Work out the finished part from the listing and answer in its coordinate system (mm). Coordinates: 2 decimals unless noted, no trailing zeros. Order: outer loops, then holes, each group sorted by start corner. A loop starts at its lowest first (then second) coordinate and runs counter-clockwise, first axis right, second up. Notation, with made-up numbers: (62, -29) -> (94, -29) arc R23 cw to (94, -2) -> close; hole circle Ø9 at (76, 83). An arc over 180 degrees is marked (long way). Use one line per item in the form item = value.
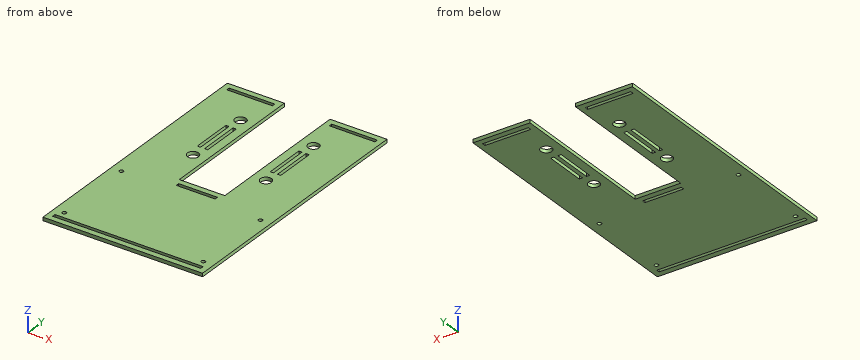
Autodesk Inventor part; units mm, degrees
ref_plane "YZ Plane" through (0, 0, 0) normal (1, 0, 0) x (0, 1, 0)
ref_plane "XZ Plane" through (0, 0, 0) normal (0, 1, 0) x (-1, 0, 0)
ref_plane "XY Plane" through (0, 0, 0) normal (0, 0, 1) x (1, 0, 0)
sketch "Sketch1" plane through (0, 0, 0) normal (0, 0, 1) x (1, 0, 0)
  line L0 (0, 0) -> (140, 0)
  line L1 (140, 0) -> (140, 232.6)
  line L2 (140, 232.6) -> (90, 232.6)
  line L3 (90, 232.6) -> (90, 100)
  line L4 (90, 100) -> (50, 100)
  line L5 (50, 100) -> (50, 232.6)
  line L6 (50, 232.6) -> (0, 232.6)
  line L7 (0, 232.6) -> (0, 0)
  line L8 (70, 100) -> (70, 0) construction
  line L9 (30, 232.2963) -> (30, 0) construction
  circle A0 centre (38, 194.6) radius 4.85
  circle A1 centre (38, 134.6) radius 4.85
  circle A2 centre (102, 194.6) radius 4.85
  circle A3 centre (102, 134.6) radius 4.85
  circle A4 centre (30, 194.6) radius 14 construction
  circle A5 centre (30, 134.6) radius 14 construction
  line L10 (5, 227.6) -> (45, 227.6)
  line L11 (45, 227.6) -> (45, 224.6)
  line L12 (45, 224.6) -> (5, 224.6)
  line L13 (5, 224.6) -> (5, 227.6)
  line L14 (53, 95) -> (87, 95)
  line L15 (87, 95) -> (87, 92)
  line L16 (87, 92) -> (53, 92)
  line L17 (53, 92) -> (53, 95)
  line L18 (5, 8) -> (135, 8)
  line L19 (135, 8) -> (135, 5)
  line L20 (135, 5) -> (5, 5)
  line L21 (5, 5) -> (5, 8)
  line L22 (135, 227.6) -> (95, 227.6)
  line L23 (95, 227.6) -> (95, 224.6)
  line L24 (95, 224.6) -> (135, 224.6)
  line L25 (135, 224.6) -> (135, 227.6)
  line L26 (30, 194.6) -> (50, 194.6) construction
  line L27 (30, 134.6) -> (50, 134.6) construction
  circle A6 centre (30, 202.6) radius 4.5
  dimension "d0" = 40
  dimension "d2" = 132.6
  dimension "d3" = 100
  dimension "d4" = 9.7
  dimension "d6" = 60
  dimension "d10" = 28
  dimension "d11" = 8
  dimension "d12" = 8
  dimension "d13" = 5
  dimension "d14" = 5
  dimension "d15" = 5
  dimension "d16" = 3
  dimension "d17" = 3
  dimension "d18" = 5
  dimension "d19" = 3
  dimension "d20" = 3
  dimension "d21" = 5
  dimension "d22" = 5
  dimension "d23" = 5
  dimension "d24" = 3
  dimension "d32" = 9
  dimension "d33" = 8
  dimension "d34" = 30
  dimension "d39" = 20
  dimension "d40" = 50
extrude "Extrusion2" add sketch "Sketch1" along normal blind 3 contours L7 L6 L5 L4 L3 L2 L1 L0 | A6
sketch "Sketch2" plane through (0, 0, 3) normal (0, 0, 1) x (1, 0, 0)
  circle A0 centre (38, 194.6) radius 4.85 construction
  line L0 (50, 232.6) -> (0, 232.6) construction
  line L1 (50, 232.6) -> (0, 232.6) construction
  line L2 (36.25, 182.6) -> (33.41, 182.6)
  line L3 (33.41, 182.6) -> (33.41, 146.6)
  line L4 (33.41, 146.6) -> (36.25, 146.6)
  line L5 (36.25, 146.6) -> (36.25, 182.6)
  line L6 (90, 100) -> (50, 100) construction
  line L7 (70, 100) -> (70, 0) construction
  line L8 (39.75, 146.6) -> (42.59, 146.6)
  line L9 (42.59, 146.6) -> (42.59, 182.6)
  line L10 (42.59, 182.6) -> (39.75, 182.6)
  line L11 (39.75, 182.6) -> (39.75, 146.6)
  line L12 (103.75, 182.6) -> (106.59, 182.6)
  line L13 (106.59, 182.6) -> (106.59, 146.6)
  line L14 (106.59, 146.6) -> (103.75, 146.6)
  line L15 (103.75, 146.6) -> (103.75, 182.6)
  line L16 (100.25, 146.6) -> (97.41, 146.6)
  line L17 (97.41, 146.6) -> (97.41, 182.6)
  line L18 (97.41, 182.6) -> (100.25, 182.6)
  line L19 (100.25, 182.6) -> (100.25, 146.6)
  line L20 (33.41, 164.6) -> (7.5179, 164.6)
  circle A1 centre (38, 134.6) radius 4.85 construction
  line L21 (38, 134.6) -> (38, 194.6)
  line L22 (38, 164.6) -> (28.9281, 164.6)
  point P0 (0, 0)
  dimension "d28" = 2.84
  dimension "d31" = 36
  dimension "d35" = 1.75
  dimension "d36" = 3.5
extrude "Extrusion3" cut sketch "Sketch2" against normal blind 3
sketch "Sketch3" plane through (0, 0, 3) normal (0, 0, 1) x (1, 0, 0)
  line L0 (5, 90) -> (135, 90)
  line L1 (135, 90) -> (135, 10)
  line L2 (135, 10) -> (5, 10)
  line L3 (5, 10) -> (5, 90)
  line L4 (5, 8) -> (135, 8) construction
  line L5 (5, 8) -> (135, 8) construction
  line L6 (135, 8) -> (135, 92) construction
  line L7 (135, 92) -> (5, 92) construction
  line L8 (5, 92) -> (5, 8) construction
  line L9 (87, 92) -> (53, 92) construction
  line L10 (135, 8) -> (135, 5) construction
  line L11 (5, 92) -> (135, 8) construction
  line L12 (5, 8) -> (135, 92) construction
  line L13 (5, 90) -> (135, 10) construction
  line L14 (5, 10) -> (135, 90) construction
  circle A0 centre (9, 86) radius 1.75
  line L15 (70, 50) -> (70, 68.0363) construction
  line L16 (70, 50) -> (82.7907, 50) construction
  circle A1 centre (131, 86) radius 1.75
  circle A2 centre (9, 14) radius 1.75
  circle A3 centre (131, 14) radius 1.75
  point P0 (0, 0)
  dimension "d37" = 130
  dimension "d38" = 80
  dimension "d41" = 3.5
  dimension "d42" = 4
  dimension "d43" = 4
extrude "Extrusion4" cut sketch "Sketch3" against normal blind 10 contours A0 | A1 | A2 | A3
equation "\"d0\" = 0.5 * marshdistance"
equation "\"d2\" = sidewallL"
equation "\"d3\" = Uthick"
equation "\"d6\" = marshmarshD"
equation "\"d34\" = marshedgeD"
equation "\"d39\" = 0.5 * Utip"
equation "\"d35\" = 0.5 * stickL"
equation "\"d36\" = stickL"
equation "\"d43\" = d42"
equation "\"thick\" = 0.5"
equation "\"lrlr\" = 19"
equation "\"lrmid\" = 19.9"
equation "\"lrdepth\" = 3.3"
equation "\"mlr\" = 16.6"
equation "\"mmid\" = 24.7"
equation "\"mdepth\" = 4.5"
equation "\"lrltotal\" = 126.6"
equation "\"mltotal\" = 126.6"
equation "\"lrbetween\" = 52.1"
equation "\"mbetween\" = 49.5"
equation "\"toler\" = 1"
equation "\"tight\" = 0.08"
equation "\"stuckw\" = 6"
equation "\"sidewallL\" = 132.6"
equation "\"heaterH\" = 117.3"
equation "\"Uthick\" = 100"
equation "\"marshmarshD\" = 60"
equation "\"marshedgeD\" = 30"
equation "\"stickL\" = 3.5"
equation "\"wireH\" = 25"
properties part number "Ushape_top"
(1) Section C-C on y = 134.6 is taken. Write down the section's boundary in (x, z).
Data:
outline = (0, 0) -> (33.15, 0) -> (33.15, 3) -> (0, 3) -> close; (42.85, 0) -> (50, 0) -> (50, 3) -> (42.85, 3) -> close; (90, 0) -> (97.15, 0) -> (97.15, 3) -> (90, 3) -> close; (106.85, 0) -> (140, 0) -> (140, 3) -> (106.85, 3) -> close
(2) Straight lines are drawn through the part: line 1 along Y through (x, z) = (64, 1.85); line 2 along Y through (x, z) = (38, 2.35); line 3 along X through (y, z) = (134, 1.6). For each, find the intervals that lie inside material, in ascending order.
Data:
line_1 = 0 to 5, 8 to 92, 95 to 100
line_2 = 0 to 5, 8 to 129.75, 139.45 to 189.75, 199.45 to 224.6, 227.6 to 232.6
line_3 = 0 to 33.19, 42.81 to 50, 90 to 97.19, 106.81 to 140
(3) Section B-B on x = 120 is taken. Write down the section's boundary in (y, z).
Data:
outline = (0, 0) -> (5, 0) -> (5, 3) -> (0, 3) -> close; (8, 0) -> (224.6, 0) -> (224.6, 3) -> (8, 3) -> close; (227.6, 0) -> (232.6, 0) -> (232.6, 3) -> (227.6, 3) -> close
(4) Section A-A on y = 173 is taken. Write down the section's boundary in (x, z).
Data:
outline = (0, 0) -> (33.41, 0) -> (33.41, 3) -> (0, 3) -> close; (36.25, 0) -> (39.75, 0) -> (39.75, 3) -> (36.25, 3) -> close; (42.59, 0) -> (50, 0) -> (50, 3) -> (42.59, 3) -> close; (90, 0) -> (97.41, 0) -> (97.41, 3) -> (90, 3) -> close; (100.25, 0) -> (103.75, 0) -> (103.75, 3) -> (100.25, 3) -> close; (106.59, 0) -> (140, 0) -> (140, 3) -> (106.59, 3) -> close
(5) This flat-tipped pin is pushed along its axis until it touches: P1, Ø0.9, axis at y = 226, z = 2, coming from the -X side. Where does it stop, or does it pass through?
Data:
P1 = 0
(6) Section D-D on z = 2.3 is taken. Count the separate pieces of the cut face and the enclosed holes in it, plus the area to 3 significant figures.
Data:
separate_pieces = 1
enclosed_holes = 16
area = 25,800 mm²
